Could you check a few things on this model? Use its own coordinates, in mm. A direction names the side the tool comes from. Give positions to 0.01 mm unless a question says otherwise; leave off trailing zeros. Write each loop counter-clockwise with the first axis right and the second up, starting at its lowest first coordinate (ties: lowest second). Pieces come first, ordered by that corner, then holes. Notation, with made-up numbers: (28.5, 6.25) - (84.5, 6.25) arc R27 ccw to (84.5, 22.25) - close; hole circle Ø1 at (-40, -15.5). An arc over 180 degrees is marked (long way). Use one line per item in the form item = value.
Autodesk Fusion 360 part; units mm, degrees
sketch "Sketch1" plane through (0, 0, 0) normal (0, 1, 0) x (1, 0, 0)
  line L0 (0, 0) -> (13.5, 0)
  line L1 (13.5, 0) -> (13.5, 17)
  line L2 (13.5, 17) -> (0, 17)
  line L3 (0, 17) -> (0, 0)
  dimension "d1" = 17
  dimension "d2" = 13.5
extrude "Extrude1" add sketch "Sketch1" along normal blind 3.5
shell "Shell1" thickness 0.8 removed faces 1 at (4.5, 0, -11.3333)
fillet "Fillet1" radius 0.8 4 edges at (6.75, 3.5, 0) (0, 3.5, -8.5) (6.75, 3.5, -17) (13.5, 3.5, -8.5)
sketch "Sketch2" plane through (0, 3.5, 0) normal (0, 1, 0) x (-1, 0, 0)
  line L0 (-12.7, -16.2) -> (-0.8, -16.2)
  line L1 (-0.8, -16.2) -> (-0.8, -0.8)
  line L2 (-0.8, -0.8) -> (-12.7, -0.8)
  line L3 (-12.7, -0.8) -> (-12.7, -16.2)
  circle A0 centre (-6.8051, -8.5) radius 5.5188
  circle A1 centre (-6.8051, -8.5) radius 4.1313
  line L4 (-6.2112, -12.8845) -> (-7.4916, -12.8845)
  line L5 (-7.4916, -12.8845) -> (-7.4916, -8.2604)
  line L6 (-7.4916, -8.2604) -> (-6.2112, -8.2604)
  line L7 (-6.2112, -8.2604) -> (-6.2112, -12.8845)
  line L8 (-4.7993, -11.3803) -> (-7.4152, -8.7643)
  line L9 (-7.4152, -8.7643) -> (-6.5099, -7.8589)
  line L10 (-6.5099, -7.8589) -> (-3.8939, -10.4749)
  line L11 (-3.8939, -10.4749) -> (-4.7993, -11.3803)
  circle A2 centre (-6.8051, -8.5) radius 0.8328
extrude "Extrude4" add sketch "Sketch2" along normal blind 0.4 contours A0 | A1 L5 L7 L8 A2 | A1 L4 L5 L7 | L5 L6 L9 L10 A2 | L5 L6 L8 L9 A2 | L7 L8 A2 | L7 L8 L10 L11 A2 | L6 L7 L9 L10 A2 | L6 L7 L8 L9 A2
1. Imagine slicing it at D-D, the plane z = -13.25. List the corners of the cut face in (x, y) for me.
Response values:
outline = (0, 0) - (0.8, 0) - (0.8, 2.7) - (12.7, 2.7) - (12.7, 0) - (13.5, 0) - (13.5, 2.7) arc R0.8 ccw to (12.7, 3.5) - (9.61, 3.5) - (9.61, 3.9) - (4, 3.9) - (4, 3.5) - (0.8, 3.5) arc R0.8 ccw to (0, 2.7) - close
2. For pin 1 (1.4 mm diameter, centred on y = 0.5, z = -5, fed in from -X); pin 2 (5 mm diameter, centred on x = 6.81, z = -8.5, fed in from -Y), each with a flat end and sliding along its axis, tell me the tip position at first contact or that it passes through.
Response values:
pin_1 = 0
pin_2 = 2.7
3. Imagine slicing it at B-B, the plane z = -2.25. List the corners of the cut face in (x, y) for me.
Response values:
outline = (0, 0) - (0.8, 0) - (0.8, 2.7) - (12.7, 2.7) - (12.7, 0) - (13.5, 0) - (13.5, 2.7) arc R0.8 ccw to (12.7, 3.5) - (0.8, 3.5) arc R0.8 ccw to (0, 2.7) - close
4. Imagine slicing it at A-A, the plane y = 0.9. List the corners of the cut face in (x, z) for me, and give its area (3 significant figures).
Response values:
outline = (0, -17) - (13.5, -17) - (13.5, 0) - (0, 0) - close; hole (0.8, -16.2) - (12.7, -16.2) - (12.7, -0.8) - (0.8, -0.8) - close
area = 46.2 mm²
5. If I drill on line 1 (Z direction, x = 12.25, y = 1.2); line 2 (X direction, y = 1.4, z = -4.5); line 3 (Y direction, x = 7, z = -9.75), over which ranges is the centre line in solid material (lowest first)? Write a range as from..to.
Response values:
line_1 = -17..-16.2, -0.8..0
line_2 = 0..0.8, 12.7..13.5
line_3 = 2.7..3.9
6. Which directions (+Z, -Z, +X, -X, +Y, -Y) give clear straight access to the entire face, cutting with the end or side of a thin tool? Please do faces 4 (the face through (13, 0, -9)), 5 (the face through (1, 3.5, -10)), 6 (the face through (7, 2.7, -9)).
Response values:
face_4 = +Z, -Z, +X, -X, -Y
face_5 = +Y
face_6 = -Y
7. If we mould it in two halves opening along X, with no side actions, what happens to faces 1 (the face through (7, 3.9, -10)), 2 (the face through (4.34, 3.7, -10.92)), 3 (the face through (13.26, 3.27, -8.62))? For each: pulls with the +X half, pulls with the -X half, needs draft (parallel to the pull), parting line crosses it, or undercut.
Response values:
face_1 = needs draft
face_2 = undercut
face_3 = pulls with the +X half
8. Imagine slicing it at C-C, the plane x = 8. List the corners of the cut face in (y, z) for me, and give its area (3 significant figures).
Response values:
outline = (0, -17) - (2.7, -17) arc R0.8 ccw to (3.5, -16.2) - (3.5, -13.89) - (3.9, -13.89) - (3.9, -12.45) - (3.5, -12.45) - (3.5, -4.55) - (3.9, -4.55) - (3.9, -3.11) - (3.5, -3.11) - (3.5, -0.8) arc R0.8 ccw to (2.7, 0) - (0, 0) - (0, -0.8) - (2.7, -0.8) - (2.7, -16.2) - (0, -16.2) - close
area = 18.8 mm²
